```python
from build123d import *

# Parameters (mm, degrees)
SKETCH1_R           = 10.5
BOSS_EXTRUDE1_DEPTH = 2.5
SKETCH3_R           = 4.5
BOSS_EXTRUDE2_DEPTH = 2
CHAMFER1_SIZE       = 2
SKETCH4_R           = 0.75
CUT_EXTRUDE1_DEPTH  = 16.058220346


with BuildPart() as part:
    # Sketch1 → Boss-Extrude1 (new body)
    with BuildSketch(Plane.XY):
        Circle(SKETCH1_R)
    extrude(amount=BOSS_EXTRUDE1_DEPTH)

    # Sketch3 → Boss-Extrude2 (add)
    with BuildSketch(Plane.XY.offset(2.5)):
        Circle(SKETCH3_R)
    extrude(amount=BOSS_EXTRUDE2_DEPTH)

    # Chamfer1
    chamfer1_edges = [part.edges().sort_by_distance(p)[0] for p in [
        (-4.5, 0, 4.5),
    ]]
    chamfer(chamfer1_edges, length=CHAMFER1_SIZE - 0.0001)  # a hair under: the kernel refuses the full size

    # Sketch4 → Cut-Extrude1 (cut, through all)
    with BuildSketch(Plane.XY.offset(2.5)):
        with Locations((0, 7)):
            Circle(SKETCH4_R)
        with Locations((7, 0)):
            Circle(SKETCH4_R)
        with Locations((0, -7)):
            Circle(SKETCH4_R)
        with Locations((-7, 0)):
            Circle(SKETCH4_R)
        with Locations((3.5, 7)):
            Circle(SKETCH4_R)
        with Locations((-3.5, 7)):
            Circle(SKETCH4_R)
        with Locations((7, -3.5)):
            Circle(SKETCH4_R)
        with Locations((7, 3.5)):
            Circle(SKETCH4_R)
        with Locations((3.5, -7)):
            Circle(SKETCH4_R)
        with Locations((-3.5, -7)):
            Circle(SKETCH4_R)
        with Locations((-7, -3.5)):
            Circle(SKETCH4_R)
        with Locations((-7, 3.5)):
            Circle(SKETCH4_R)
    extrude(amount=-CUT_EXTRUDE1_DEPTH, mode=Mode.SUBTRACT)


solid = part.part
```
Check sheet for the modelled part. Datum: model origin and axes. Units: mm. A direction names the side the tool comes from. Coordinates: 2 decimals unless noted, no trailing zeros. Order: outer loops, then holes, each group sorted by start corner. A loop starts at its lowest first (then second) coordinate and runs counter-clockwise, first axis right, second up. Notation, with made-up numbers: M 12.5,80.25 L 64.5,80.25 A22 ccw 64.5,103.25 Z; hole C 74,-16 d5. An arc over 180 degrees is marked long. Write each question's results on one line, items separated by ' | '. Start each with the question number.
1. Material ranges on probe 1 along Y at (x, z) = (0, 0.7); probe 2 along Y at (x, z) = (-4, 2.15); probe 3 along Y at (x, z) = (7, 1), recorded low to high.
2. Cross-section at D-D on y = 7.5. Record the cut outline in (x, z), and give its area (3 significant figures).
3. Access from +Z, -Z, +X, -X, +Y, -Y to the whole of each face (thin tool, end or side, straight path). Record for faces 1 (the face through (-7.595, 3.044, 1.268)), 2 (the face through (5, 0, 2.5)).
4. Cross-section at C-C on x = 7. Record the cut outline in (y, z), and give its area (3 significant figures).
5. Go/stop test with flat-tipped pins: P1, Ø1.2, axis at x = -7, y = 3.5, coming from the -Z side; P2, Ø2, axis at x = -6, y = 0.5, coming from the +Z side; P3, Ø1.5, axis at y = -2, z = 1, coming from the +X side. Record where each tip stops, or that it passes through.
6. Cross-section at A-A on y = 0. State how many separate pieces and enclosed holes the cut face has, and give its area (3 significant figures).
7. Mould release check, pull along Y, two halves, no side actions. Record for faces 3 (the face through (2.75, 7.03, 1.27)), 4 (the face through (0, 0, 4.5)), 5 (the face through (-3, 0, 4)): +Y half, -Y half, draft (parallel to the pull), parting line (faces both ways), or undercut.
Checks:
1) probe 1: y = -10.5 to -7.75, -6.25 to 6.25, 7.75 to 10.5 | probe 2: y = -9.71 to -7.56, -6.44 to 6.44, 7.56 to 9.71 | probe 3: y = -7.83 to -4.25, -2.75 to -0.75, 0.75 to 2.75, 4.25 to 7.83
2) outline: M -7.35,0 L -4.06,0 L -4.06,2.5 L -7.35,2.5 Z; M -2.94,0 L -0.56,0 L -0.56,2.5 L -2.94,2.5 Z; M 0.56,0 L 2.94,0 L 2.94,2.5 L 0.56,2.5 Z; M 4.06,0 L 7.35,0 L 7.35,2.5 L 4.06,2.5 Z | area: 28.4 mm²
3) face 1: +Z, -Z | face 2: +Z
4) outline: M -7.83,0 L -4.25,0 L -4.25,2.5 L -7.83,2.5 Z; M -2.75,0 L -0.75,0 L -0.75,2.5 L -2.75,2.5 Z; M 0.75,0 L 2.75,0 L 2.75,2.5 L 0.75,2.5 Z; M 4.25,0 L 7.83,0 L 7.83,2.5 L 4.25,2.5 Z | area: 27.9 mm²
5) P1: passes through | P2: stops at z = 2.5 | P3: stops at x = 10.43
6) separate pieces: 3 | enclosed holes: 0 | area: 59.0 mm²
7) face 3: undercut | face 4: draft | face 5: parting line
